Check sheet for the modelled part. Datum: model origin and axes. Units: mm. A direction names the side the tool comes from. Round coordinates to 2 decimals unless told otherwise and drop trailing zeros. Order: outer loops, then holes, each group sorted by start corner. A loop starts at its lowest first (then second) coordinate and runs counter-clockwise, first axis right, second up. Notation, with made-up numbers: (25, 27) -> (77, 27) arc R27 ccw to (77, 56) -> close; hole circle Ø4 at (65.5, 48.5). An arc over 180 degrees is marked (long way). Answer in a Markdown table with one row per item. Add a question column.
1. Sectioned sample at A-A, the plane y = 1.5. Count the separate pieces of the cut face and the enclosed holes in it, then the cut area to 3 significant figures.
2. Sectioned sample at B-B, the plane x = 122. Record the boundary of the cut face in (y, z).
3. Draft check along Z on faces 1 (the flat face through (177, 2, -148.48)), 2 (the cylindrical face through (108.785, 2.465, -77.327)), 3 (the flat face through (99.93, 2, -139)). Enter one of: +Z half, -Z half, draft (parallel to the pull), parting line (faces both ways), or undercut.
4. Depth check by flat-ended pin: P1, Ø1.8, axis at x = 66.18, z = -4, coming from the +Y side; P2, Ø1.5, axis at x = 110, y = 1.5, coming from the -Z side. Enter the tip coordinate at first touch or a pass-through.
5. Material ranges on L1, parallel to Z at x = 223.86, y = 2.35; L2, parallel to X at y = 3.55, z = -74.24; L3, parallel to X at y = 0.7, z = -135, recorded low to high. Write a range as from..to.
6. Access from +Z, -Z, +X, -X, +Y, -Y to the whole of each face (thin tool, end or side, straight path). Record for faces 4 (the flat face through (127.93, 2, -138)), 5 (the flat face through (120.99, 2.46, -77.12)), 6 (the flat face through (49, 2, -148.48)).
```python
from build123d import *

# Parameters (mm, degrees)
SKETCH1_R           = 1.5
BOSS_EXTRUDE1_DEPTH = 5


with BuildPart() as part:
    # Sketch1 → Boss-Extrude1 (new body)
    with BuildSketch(Plane(origin=(0, 0, 0), x_dir=(1, 0, 0), z_dir=(0, 1, 0))):
        Polygon((0, 0), (0, 148.48), (99.93, 148.48), (99.93, 128.48), (127.93, 128.48), (127.93, 148.48), (227.86, 148.48), (227.86, 0), align=None)
        with Locations(Location((223.86, 74.24, 0), (0, 0, 270))):
            Circle(SKETCH1_R, mode=Mode.SUBTRACT)
        with Locations(Location((4, 74.24, 0), (0, 0, 90))):
            Circle(SKETCH1_R, mode=Mode.SUBTRACT)
        with Locations(Location((66.18, 4, 0), (0, 0, 270))):
            Circle(SKETCH1_R, mode=Mode.SUBTRACT)
        with Locations(Location((161.68, 4, 0), (0, 0, 270))):
            Circle(SKETCH1_R, mode=Mode.SUBTRACT)
        with Locations(Location((161.68, 144.48, 0), (0, 0, 270))):
            Circle(SKETCH1_R, mode=Mode.SUBTRACT)
        with Locations(Location((66.18, 144.48, 0), (0, 0, 270))):
            Circle(SKETCH1_R, mode=Mode.SUBTRACT)
        with Locations(Location((223.86, 4, 0), (0, 0, 270))):
            Circle(SKETCH1_R, mode=Mode.SUBTRACT)
        with Locations(Location((4, 4, 0), (0, 0, 90))):
            Circle(SKETCH1_R, mode=Mode.SUBTRACT)
        with Locations(Location((4, 144.48, 0), (0, 0, 270))):
            Circle(SKETCH1_R, mode=Mode.SUBTRACT)
        with Locations(Location((223.86, 144.48, 0), (0, 0, 90))):
            Circle(SKETCH1_R, mode=Mode.SUBTRACT)
        with BuildLine():
            Line((124.972729238, 74.848802076), (116.902729238, 79.451802076))
            ThreePointArc((116.902729238, 79.451802076), (108.718197924, 77.212729238), (110.957270762, 69.028197924))
            Line((110.957270762, 69.028197924), (119.027270762, 64.425197924))
            ThreePointArc((119.027270762, 64.425197924), (127.211802076, 66.664270762), (124.972729238, 74.848802076))
        make_face(mode=Mode.SUBTRACT)
    extrude(amount=BOSS_EXTRUDE1_DEPTH)


solid = part.part
```
Answer key:
| question | item | result |
|---|---|---|
| 1 | separate pieces | 1 |
| 1 | enclosed holes | 11 |
| 1 | area | 33,000 mm² |
| 2 | outline | (0, -128.48) -> (5, -128.48) -> (5, -76.54) -> (0, -76.54) -> close; (0, -63.64) -> (5, -63.64) -> (5, 0) -> (0, 0) -> close |
| 3 | face 1 | -Z half |
| 3 | face 2 | undercut |
| 3 | face 3 | draft |
| 4 | P1 | passes through |
| 4 | P2 | stops at z = -128.48 |
| 5 | L1 | z = -148.48..-145.98, -142.98..-75.74, -72.74..-5.5, -2.5..0 |
| 5 | L2 | x = 0..2.5, 5.5..107.93, 125.85..222.36, 225.36..227.86 |
| 5 | L3 | x = 0..99.93, 127.93..227.86 |
| 6 | face 4 | -Z, +Y, -Y |
| 6 | face 5 | +Y, -Y |
| 6 | face 6 | -Z, +X, -X, +Y, -Y |
